Model file for the job. Use its own axes, mm. Face numbers are marked on the shaded views. A direction names the side the tool comes from. Round coordinates to 2 decimals unless told otherwise and drop trailing zeros. Loops run counter-clockwise (first coordinate to the right, second up) from the corner with the lowest first, then second, coordinate; pieces in that order, holes last. Notation, with made-up numbers: M -12.5,63 L 29.5,63 A12 cw 29.5,76 Z; hole C 22,-35 d4. An arc over 180 degrees is marked long. Use a Markdown table: item, result. Add a question column.
Item 1: Wall check: L1, parallel to Y at x = -1.25, z = -5; L2, parallel to X at y = 6, z = -16.5; L3, parallel to Z at x = 9.5, y = 2.75. Give the ranges that are in metal, low to high. Write a range as from..to.
Item 2: Saw through at D-D on x = 1.25. Write the cut outline in (y, z), then the cut area to 3 significant figures.
Item 3: Tool access for the marked faces 1 and 2: list every direction of +Z, -Z, +X, -X, +Y, -Y with a clear straight run to the whole face (end or side of a thin tool).
Item 4: Saw through at C-C on y = 4. Write the cut outline in (x, z).
Item 5: Saw through at B-B on x = 5. Write the cut outline in (y, z), then the cut area to 3 significant figures.
Item 6: Two-plate mould, pull along Y, no slides. Class the marked faces 3, 4, 5 and 6: +Y half, -Y half, draft (parallel to the pull), parting line (faces both ways), or undercut.
Item 7: Saw through at A-A on z = -5. Write the cut outline in (x, y).
Item 8: Pin check, flat tips, straight feed: P1, Ø4, axis at y = 5, z = -14.5, coming from the +X side; P2, Ø4.5, axis at x = 15, y = 4, coming from the -Z side. Stop position of each tip, or through.
```python
from build123d import *

# Parameters (mm, degrees)
BOSS_EXTRUDE1_DEPTH = 8
SKETCH2_R           = 2
CUT_EXTRUDE1_DEPTH  = 8
SKETCH3_R           = 2
CUT_EXTRUDE2_DEPTH  = 8
FILLET3_R           = 2


with BuildPart() as part:
    # Sketch1 → Boss-Extrude1 (new body)
    with BuildSketch(Plane(origin=(0, 0, 0), x_dir=(1, 0, 0), z_dir=(0, 1, 0))):
        Polygon((0, 20), (0, 0), (20, 0), (20, -2), (-2, -2), (-2, 20), align=None)
    extrude(amount=BOSS_EXTRUDE1_DEPTH)

    # Sketch2 → Cut-Extrude1 (cut)
    with BuildSketch(Plane(origin=(0, 0, 0), x_dir=(-1, 0, 0), z_dir=(0, 0, -1))):
        with Locations((-15, 4)):
            Circle(SKETCH2_R)
        with Locations((-5, 4)):
            Circle(SKETCH2_R)
    extrude(amount=-CUT_EXTRUDE1_DEPTH, mode=Mode.SUBTRACT)

    # Sketch3 → Cut-Extrude2 (cut)
    with BuildSketch(Plane(origin=(0, 0, 0), x_dir=(0, 0, -1), z_dir=(1, 0, 0))):
        with Locations((5, 4)):
            Circle(SKETCH3_R)
        with Locations((15, 4)):
            Circle(SKETCH3_R)
    extrude(amount=-CUT_EXTRUDE2_DEPTH, mode=Mode.SUBTRACT)

    # Fillet3
    fillet3_edges = [part.edges().sort_by_distance(p)[0] for p in [
        (-2, 4, 2),
    ]]
    fillet(fillet3_edges, radius=FILLET3_R)


solid = part.part
```
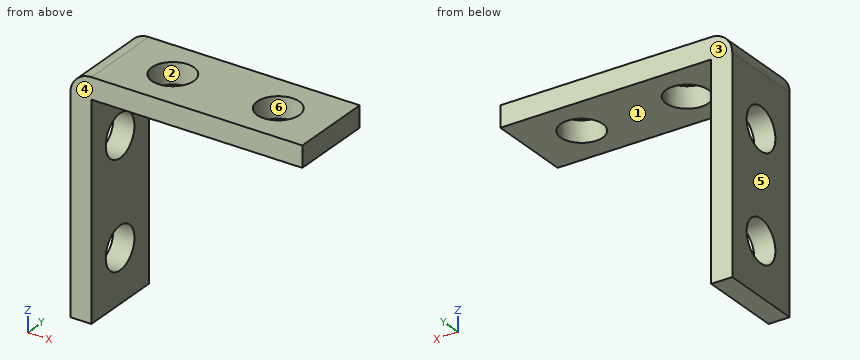
Entries:
| question | item | result |
|---|---|---|
| 1 | L1 | 0..2, 6..8 |
| 1 | L2 | -2..0 |
| 1 | L3 | 0..2 |
| 2 | outline | M 0,0 L 8,0 L 8,2 L 0,2 Z |
| 2 | area | 16.0 mm2 |
| 3 | face 1 | -Z, +X, +Y, -Y |
| 3 | face 2 | +Z, -Z |
| 4 | outline | M -2,-20 L 0,-20 L 0,-17 L -2,-17 Z; M -2,-13 L 0,-13 L 0,-7 L -2,-7 Z; M -2,-3 L 0,-3 L 0,0 L 3,0 L 3,2 L 0,2 A2 ccw -2,0 Z; M 7,0 L 13,0 L 13,2 L 7,2 Z; M 17,0 L 20,0 L 20,2 L 17,2 Z |
| 5 | outline | M 0,0 L 2,0 L 2,2 L 0,2 Z; M 6,0 L 8,0 L 8,2 L 6,2 Z |
| 5 | area | 8.00 mm2 |
| 6 | face 3 | +Y half |
| 6 | face 4 | -Y half |
| 6 | face 5 | draft |
| 6 | face 6 | undercut |
| 7 | outline | M -2,0 L 0,0 L 0,2 L -2,2 Z; M -2,6 L 0,6 L 0,8 L -2,8 Z |
| 8 | P1 | x = 0 |
| 8 | P2 | z = 0 |
